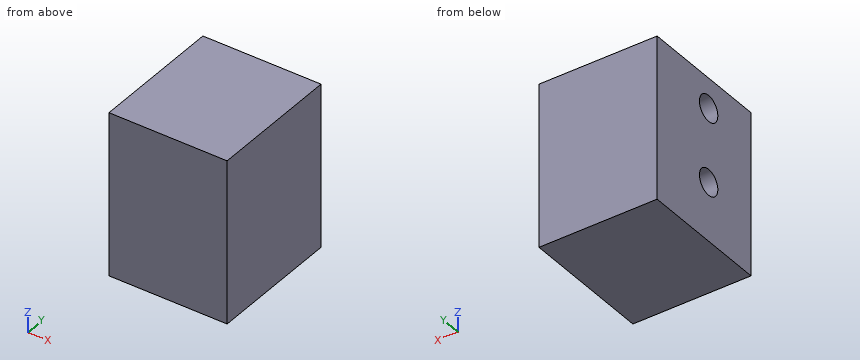
from build123d import *

# Parameters (mm, degrees)
SKETCH1_W                   = 55.233155238
SKETCH1_H                   = 45
BOSS_EXTRUDE1_DEPTH         = 40
M10X1_25_TAPPED_HOLE1_D     = 8.8
M10X1_25_TAPPED_HOLE1_DEPTH = 11.75
M10X1_25_TAPPED_HOLE1_TIP   = 2.643786724


with BuildPart() as part:
    # Sketch1 → Boss-Extrude1 (new body)
    with BuildSketch(Plane(origin=(-82.778181514, 0, 0), x_dir=(0, 0, -1), z_dir=(1, 0, 0))):
        with Locations((-566.428701217, 22.5)):
            Rectangle(SKETCH1_W, SKETCH1_H)
    extrude(amount=BOSS_EXTRUDE1_DEPTH)

    # M10x1.25 Tapped Hole1
    with Locations(Plane.ZY.offset(82.778181514)):
        with Locations((583.767961031, 20.315155656), (558.767961031, 20.315155656)):
            Hole(M10X1_25_TAPPED_HOLE1_D / 2, depth=M10X1_25_TAPPED_HOLE1_DEPTH)
            with Locations((0, 0, -(M10X1_25_TAPPED_HOLE1_DEPTH + M10X1_25_TAPPED_HOLE1_TIP / 2))):  # 118° drill point
                Cone(0, M10X1_25_TAPPED_HOLE1_D / 2, M10X1_25_TAPPED_HOLE1_TIP, mode=Mode.SUBTRACT)


solid = part.part
For this review, take the finished solid that the model builds, in its own axes (mm). Give positions to 0.01 mm unless a question says otherwise; leave off trailing zeros. Loops run counter-clockwise (first coordinate to the right, second up) from the corner with the lowest first, then second, coordinate; pieces in that order, holes last. Notation, with made-up numbers: M 39.25,10 L 96.25,10 A16 cw 96.25,20 Z; hole C 16,-11 d2. An arc over 180 degrees is marked long. Answer as a JSON object with one key per item and string values. Group by question number.
Q1. Add section A-A on x = -73. Give the boundary of the cut face in (y, z), and give its area (3 significant figures).
Q2. For probe 1 along Z at (x, y) = (-75, 17.5); probe 2 along Z at (x, y) = (-79, 23), list the stretches that pass through material, from the lowest coordinate up. Write a range as [from, to].
Q3. Insertion check: P1, Ø5.5, axis at y = 20.32, z = 583.77, coming from the -X side; P2, Ø8, axis at y = 20.32, z = 558.77, coming from the -X side. Each pin has a flat end and moves straight along its axis. Give the tip position at first contact, or say it passes through.
Checked values:
{
 "1": {"outline": "M 0,538.81 L 45,538.81 L 45,594.05 L 0,594.05 Z; hole C 20.32,558.77 d8.8; hole C 20.32,583.77 d8.8", "area": "2,360 mm²"},
 "2": {"probe 1": "[538.81, 555.39], [562.15, 580.39], [587.15, 594.05]", "probe 2": "[538.81, 555.28], [562.25, 580.28], [587.25, 594.05]"},
 "3": {"P1": "x = -70.04", "P2": "x = -70.79"}
}
